For this review, take the finished solid that the model builds, in its own axes (mm). Give positions to 0.01 mm unless a question says otherwise; leave off trailing zeros. Order: outer loops, then holes, each group sorted by start corner. A loop starts at its lowest first (then second) coordinate and runs counter-clockwise, first axis right, second up. Notation, with made-up numbers: (75, 52.25) -> (103, 52.25) arc R6 cw to (103, 60.25) -> close; hole circle Ø7 at (37, 70.5). An arc over 180 degrees is marked (long way). Return JSON: item names as keys, results as strings. Group by question number.
1) Insertion check: P1, Ø8, axis at y = -12, z = 22.5, coming from the -X side; P2, Ø3, axis at x = 51, y = -19, coming from the -Z side; P3, Ø10, axis at y = -23, z = -17.5, coming from the +X side; P4, Ø1.5, axis at x = 17.5, y = -6, coming from the -Z side. Each pin has a flat end and moves straight along its axis. Give the tip position at first contact, or say it passes through.
2) Add section C-C (y = -4.25). Give the boundary of the cut face in (x, z).
3) To check wall thickness, follow line 1 along X through (y, z) = (-12, -28); line 2 along Z through (x, y) = (52.5, -13); line 3 along X through (y, z) = (-3.5, 2.5). State the ranges of each line that lie inside material, in increasing order.
4) Add section D-D (y = -18.5). Give the boundary of the cut face in (x, z), then the cut area to 3 significant figures.
from build123d import *

# Parameters (mm, degrees)
F0_W     = 101.6
F0_H     = 101.6
F1_DEPTH = 25.4
F2_R     = 12.69999


# Not quite as in the source:
# - a fillet or chamfer is up to 0.001 mm smaller than in the source, because OpenCascade refuses the exact size


with BuildPart() as f1:
    # F0 (on Front) → F1 (new body)
    with BuildSketch(Plane.XZ):
        with Locations((12.5491575718, -14.5562545776)):
            Rectangle(F0_W, F0_H)
    extrude(amount=F1_DEPTH)

    # F2 (radius 12.7 in the source; OpenCascade refuses exactly that, so slightly less here)
    f2_edges = [f1.edges().sort_by_distance(p)[0] for p in [
        (12.549158, 0, -65.356255),
        (63.349158, 0, -14.556255),
        (12.549158, 0, 36.243745),
        (-38.250842, 0, -14.556255),
        (12.549158, -25.4, -65.356255),
        (63.349158, -25.4, -14.556255),
        (12.549158, -25.4, 36.243745),
        (-38.250842, -25.4, -14.556255),
    ]]
    fillet(f2_edges, radius=F2_R)


solid = f1.part
Evaluation:
{
 "1": {"P1": "x = -38.25", "P2": "z = -64.41", "P3": "x = 62.19", "P4": "z = -63.88"},
 "2": {"outline": "(-35.03, -62.14) -> (60.13, -62.14) -> (60.13, 33.02) -> (-35.03, 33.02) -> close"},
 "3": {"line 1": "-38.23 to 63.33", "line 2": "-65.35 to 36.24", "line 3": "-34.31 to 59.4"},
 "4": {"outline": "(-36.85, -63.95) -> (61.95, -63.95) -> (61.95, 34.84) -> (-36.85, 34.84) -> close", "area": "9,760 mm^2"}
}
